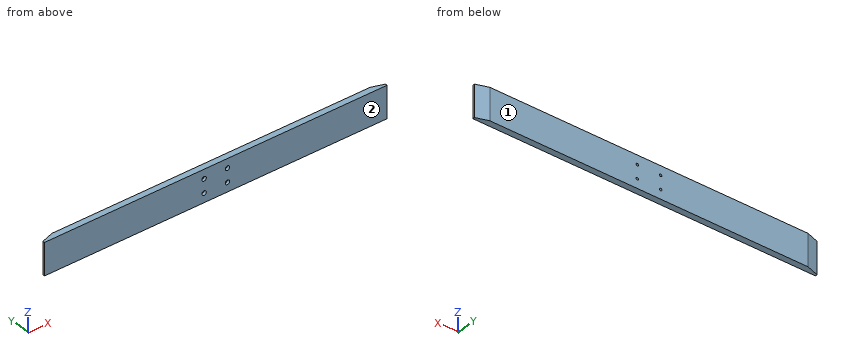
from build123d import *

# Parameters (mm, degrees)
F0_W           = 850
F0_H           = 80
F1_DEPTH       = 7.5
F3_D           = 6
F3_CBORE_D     = 11
F3_CBORE_DEPTH = 7
F4_D           = 0.1
F6_DEPTH       = 80.001


with BuildPart() as f1:
    # F0 (on Front) → F1 (new body, symmetric)
    with BuildSketch(Plane.XZ):
        Rectangle(F0_W, F0_H)
    extrude(amount=F1_DEPTH, both=True)

    # F3 (through all)
    with Locations(Plane.XZ.offset(7.5)):
        with Locations((-29, 17), (29, 17), (29, -17), (-29, -17)):
            CounterBoreHole(F3_D / 2, F3_CBORE_D / 2, F3_CBORE_DEPTH)

    # F4 (through all)
    with Locations(Plane.XZ.offset(7.5)):
        with Locations((0, 0)):
            Hole(F4_D / 2)

    # F5 (on face) → F6 (cut, through all)
    with BuildSketch(Plane.XY.offset(40)):
        Polygon((-395, 7.5), (-425, 7.5), (-425, -2.5), align=None)
        Polygon((425, 7.5), (395, 7.5), (425, -2.5), align=None)
    extrude(amount=-F6_DEPTH, mode=Mode.SUBTRACT)


solid = f1.part
The listing builds one solid part. Answer for the finished solid, in the listing's coordinates (mm). Face numbers are marked on the shaded views. Coordinates: 2 decimals unless noted, no trailing zeros. Loops run counter-clockwise (first coordinate to the right, second up) from the corner with the lowest first, then second, coordinate; pieces in that order, holes last. Notation, with made-up numbers: (-20, 2.25) -> (-5, 2.25) arc R23 cw to (-5, 18.25) -> close; hole circle Ø3 at (25.5, 18). An arc over 180 degrees is marked (long way). Write item = value, one per line. Start each with the question number.
1) A cutting plane is placed at B-B (z = -32). Give the vertices of the cut face in (x, y).
2) Given pin 1 Ø5.5 at (x, z) = (-30.5, 18.5) entering from -Y; pin 2 Ø9 at (x, z) = (-29, 17) entering from +Y; pin 3 Ø5.5 at (x, z) = (29, -17) entering from -Y, each flat-ended and moving along its own axis, determine where each tip first touches the part or whether it passes through.
3) The mould has two halves that part along Y. Classify the marked faces 1 and 2: released by +Y, released by -Y, zero draft, split by the parting line, or undercut.
4) Straight lines are drawn through the part: line 1 (X direction, y = -4.5, z = 16.5); line 2 (Z direction, x = 29, y = -5); line 3 (X direction, y = -5, z = 14). For each, find the intervals that lie inside material, in ascending order. Write a range as from..to.
Responses:
q1.outline = (-425, -7.5) -> (425, -7.5) -> (425, -2.5) -> (395, 7.5) -> (-395, 7.5) -> (-425, -2.5) -> close
q2.pin_1 = -0.5
q2.pin_2 = 7.5
q2.pin_3 = through
q3.face_1 = released by +Y
q3.face_2 = released by -Y
q4.line_1 = -425..-34.48, -23.52..23.52, 34.48..425
q4.line_2 = -40..-22.5, -11.5..11.5, 22.5..40
q4.line_3 = -425..-33.61, -24.39..24.39, 33.61..425
